Autodesk Inventor part; units mm, degrees
ref_plane "YZ Plane" through (0, 0, 0) normal (1, 0, 0) x (0, 1, 0)
ref_plane "XZ Plane" through (0, 0, 0) normal (0, 1, 0) x (-1, 0, 0)
ref_plane "XY Plane" through (0, 0, 0) normal (0, 0, 1) x (1, 0, 0)
sketch "スケッチ1" plane through (0, 0, 0) normal (0, 0, 1) x (1, 0, 0)
  circle A0 centre (0, 0) radius 4
  dimension "d13" = 8
extrude "押し出し1" add sketch "スケッチ1" along normal blind 77
sketch "スケッチ2" plane through (0, 0, 77) normal (0, 0, 1) x (1, 0, 0)
  point P0 (0, 0)
  point P1 (0, 0)
hole "穴1" at (0, 0, 77) direction (0, 0, -1) diameter 3.242 end through all
chamfer "面取り1" distance 0.2 angle 45 4 edges at (0, 1.621, 77) (0, 1.621, 0) (-4, 0, 77) (-4, 0, 0)
properties part number "ARF-4_2" material "鋼、炭素鋼"
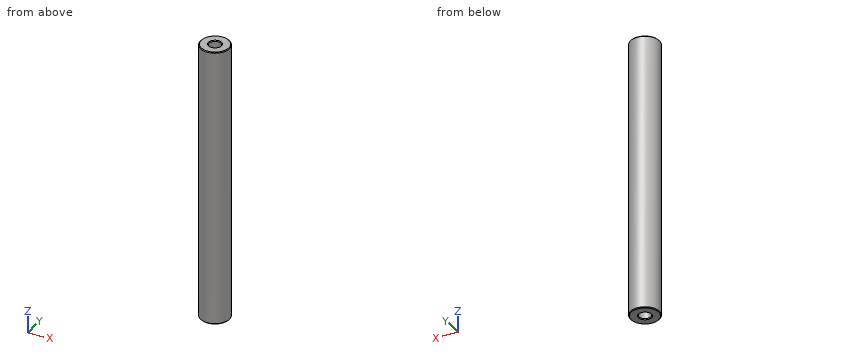
Work out the finished part from the listing and answer in its coordinate system (mm). Give positions to 0.01 mm unless a question says otherwise; leave off trailing zeros. Loops run counter-clockwise (first coordinate to the right, second up) from the corner with the lowest first, then second, coordinate; pieces in that order, holes last. Notation, with made-up numbers: M 89.5,15 L 134.5,15 A20 ccw 134.5,54 Z; hole C 64.5,50 d3. An arc over 180 degrees is marked long. Use CSV: the item, a comma, the result in double quotes.
1) Find section C-C on z = 54.5. Write down the section's boundary in (x, y), plus the area to 3 significant figures.
Answer:
outline,"C 0,0 d8; hole C 0,0 d3.24"
area,"42.0 mm^2"
2) Consider L1, parallel to Y at x = 0, z = 40; L2, parallel to X at y = -0.5, z = 46.5; L3, parallel to Z at x = 2, y = -3.25. Determine where each line is inside the solid, lowest interval first.
Answer:
L1,"-4 to -1.62, 1.62 to 4"
L2,"-3.97 to -1.54, 1.54 to 3.97"
L3,"0.02 to 76.98"
3) Given P1, Ø3, axis at x = 2.5, z = 9.5, coming from the +Y side; P2, Ø3, axis at y = -2.5, z = 15, coming from the +X side, each flat-ended and moving along its own axis, determine where each tip first touches the part or whether it passes through.
Answer:
P1,"y = 3.87"
P2,"x = 3.87"
4) Find section A-A on y = 0. Write down the section's boundary in (x, z).
Answer:
outline,"M -4,0.2 L -3.8,0 L -1.82,0 L -1.62,0.2 L -1.62,76.8 L -1.82,77 L -3.8,77 L -4,76.8 Z; M 1.62,0.2 L 1.82,0 L 3.8,0 L 4,0.2 L 4,76.8 L 3.8,77 L 1.82,77 L 1.62,76.8 Z"
